Build history of the part. All positions in model axes, mm. Round coordinates to 2 decimals unless told otherwise and drop trailing zeros. Write each loop counter-clockwise with the first axis right and the second up, starting at its lowest first coordinate (ties: lowest second). Pieces come first, ordered by that corner, then holes.
Item 1: Drop flat-ended pins along their axis: pin 1 Ø8 at (x, y) = (49, 65) entering from +Z; pin 2 Ø15 at (x, y) = (-48.5, -96.5) entering from +Z; pin 3 Ø3.5 at (x, z) = (49, 9) entering from -Y. Give the stop position or say it passes through.
Item 2: Band-saw the part on C-C, the plane z = 12. Write the cut outline in (x, y), then the cut area to 3 significant figures.
Item 3: Band-saw the part on D-D, the plane x = -43.5. Write the cut outline in (y, z) (3 decimals), then the cut area to 3 significant figures.
Item 4: Band-saw the part on B-B, the plane y = 37. Write the cut outline in (x, z) (1 decimal).
Item 5: Band-saw the part on A-A, the plane x = 69. Write the cut outline in (y, z) (3 decimals).
Item 6: Wall check: probe 1 along X at (y, z) = (-30.5, 4.25); probe 2 along Y at (x, z) = (9.5, 3.5); probe 3 along Z at (x, y) = (32, -76) (3 decimals). Give the ranges that are in metal, low to high.
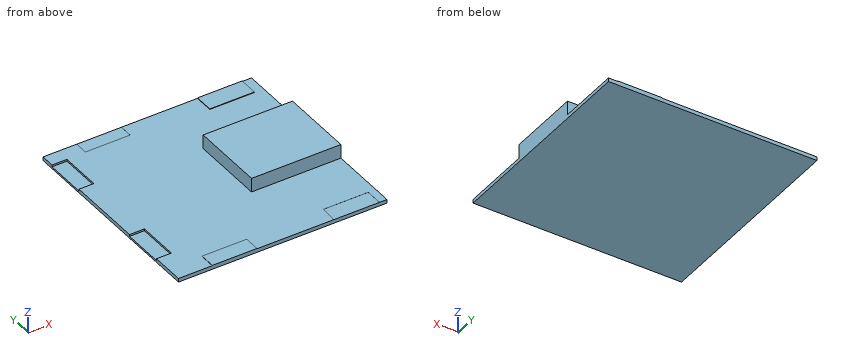
```python
from build123d import *

# Parameters (mm, degrees)
F1_DEPTH = 3.175
F0_W     = 12.7
F0_H     = 35.3568
F0_H_2   = 35.3450775146
F2_DEPTH = 1.5875
F0_W_2   = 76.2
F0_H_3   = 63.5
F3_DEPTH = 1.5875
F0_W_3   = 38.1
F0_H_4   = 13.5492910243
F4_DEPTH = 3.41914
F5_DEPTH = 3.13733
F0_H_5   = 11.4938615345
F6_DEPTH = 3.12486
F0_H_6   = 16.1283126556
F7_DEPTH = 3.5988
F8_DEPTH = 13.55152


with BuildPart() as f1:
    # F0 (on Top) → F1 (new body)
    with BuildSketch(Plane.XY):
        Polygon((-67.3727616668, 74.7556908511), (-96.1277933359, 74.7556908511), (-96.1277933359, 62.904787178), (-83.4277933359, 62.904787178), (-83.4277933359, 27.547987178), (-96.1277933359, 27.547987178), (-96.1277933359, -38.7955904007), (-83.4277933359, -38.7955904007), (-83.4277933359, -74.1406679153), (-96.1277933359, -74.1406679153), (-96.1277933359, -103.0443091489), (-67.2837272286, -103.0443091489), (-67.2837272286, -89.4950181246), (-29.1837272286, -89.4950181246), (-29.1837272286, -103.0443091489), (36.3641157746, -103.0443091489), (37.1394492686, -88.3632972836), (75.2394492686, -88.3632972836), (75.2394492686, -103.0443091489), (81.6722066641, -103.0443091489), (81.6722066641, -42.5480678678), (5.4722066641, -42.5480678678), (5.4722066641, 20.9519321322), (81.6722066641, 20.9519321322), (81.6722066641, 74.7556908511), (73.7083251536, 74.7556908511), (73.7083251536, 58.6273781955), (35.6083251536, 58.6273781955), (35.6083251536, 74.7556908511), (-29.2727616668, 74.7556908511), (-29.2727616668, 63.2618293166), (-67.3727616668, 63.2618293166), align=None)
    extrude(amount=F1_DEPTH)

    # F0 (on Top) → F2 (join)
    with BuildSketch(Plane.XY):
        with Locations((-89.7777933359, 45.226387178)):
            Rectangle(F0_W, F0_H)
        with Locations((-89.7777933359, -56.468129158)):
            Rectangle(F0_W, F0_H_2)
    extrude(amount=F2_DEPTH)

    # F0 (on Top) → F3 (join)
    with BuildSketch(Plane.XY):
        with Locations((43.5722066641, -10.7980678678)):
            Rectangle(F0_W_2, F0_H_3)
    extrude(amount=F3_DEPTH)

    # F0 (on Top) → F4 (join)
    with BuildSketch(Plane.XY):
        with Locations((-48.2337272286, -96.2696636367)):
            Rectangle(F0_W_3, F0_H_4)
    extrude(amount=F4_DEPTH)

    # F0 (on Top) → F5 (join)
    with BuildSketch(Plane.XY):
        Polygon((37.1394492686, -88.3632972836), (36.3641157746, -103.0443091489), (75.2394492686, -103.0443091489), (75.2394492686, -88.3632972836), align=None)
    extrude(amount=F5_DEPTH)

    # F0 (on Top) → F6 (join)
    with BuildSketch(Plane.XY):
        with Locations((-48.3227616668, 69.0087600839)):
            Rectangle(F0_W_3, F0_H_5)
    extrude(amount=F6_DEPTH)

    # F0 (on Top) → F7 (join)
    with BuildSketch(Plane.XY):
        with Locations((54.6583251536, 66.6915345233)):
            Rectangle(F0_W_3, F0_H_6)
    extrude(amount=F7_DEPTH)

    # F8 (add): a face of the model
    f8_faces = [f1.faces().sort_by_distance(p)[0] for p in [
        (43.5722066641, -10.7980678678, 1.5875),
    ]]
    extrude(f8_faces, amount=F8_DEPTH)


solid = f1.part
```
Results:
1. pin 1: stops at z = 3.6
1. pin 2: stops at z = 3.42
1. pin 3: stops at y = -42.55
2. outline: (5.47, -42.55) - (81.67, -42.55) - (81.67, 20.95) - (5.47, 20.95) - close
2. area: 4,840 mm2
3. outline: (-103.044, 0) - (74.756, 0) - (74.756, 3.125) - (63.262, 3.125) - (63.262, 3.175) - (-89.495, 3.175) - (-89.495, 3.419) - (-103.044, 3.419) - close
3. area: 567 mm2
4. outline: (-96.1, 0) - (81.7, 0) - (81.7, 3.2) - (-83.4, 3.2) - (-83.4, 1.6) - (-96.1, 1.6) - close
5. outline: (-103.044, 0) - (74.756, 0) - (74.756, 3.599) - (58.627, 3.599) - (58.627, 3.175) - (20.952, 3.175) - (20.952, 15.139) - (-42.548, 15.139) - (-42.548, 3.175) - (-88.363, 3.175) - (-88.363, 3.137) - (-103.044, 3.137) - close
6. probe 1: x = 5.47 to 81.67
6. probe 2: y = -42.55 to 20.95
6. probe 3: z = 0 to 3.175
